from build123d import *

# Parameters (mm, degrees)
CROQUIS1_R              = 4
SALIENTE_EXTRUIR1_DEPTH = 12
CORTAR_EXTRUIR2_DEPTH   = 8
CORTAR_EXTRUIR3_START   = -2.5000001
CORTAR_EXTRUIR3_DEPTH   = 4.0000001


# Read off the part's stored shape, not the designer's step: Cortar-Extruir3
with BuildPart() as part:
    # Croquis1 → Saliente-Extruir1 (new body)
    with BuildSketch(Plane.XY):
        Circle(CROQUIS1_R)
    extrude(amount=SALIENTE_EXTRUIR1_DEPTH)

    # Croquis1<5> → Cortar-Extruir2 (cut)
    with BuildSketch(Plane.XY):
        with BuildLine():
            Line((-1.322875656, 1.5), (1.322875656, 1.5))
            ThreePointArc((1.322875656, 1.5), (0, -2), (-1.322875656, 1.5))
        make_face()
    extrude(amount=CORTAR_EXTRUIR2_DEPTH, mode=Mode.SUBTRACT)

    # Cortar-Extruir3 outline → Cortar-Extruir3 (cut)
    with BuildSketch(Plane.XZ.offset(-1.5).offset(CORTAR_EXTRUIR3_START)):
        with BuildLine():
            ThreePointArc((2, 5), (0, 7), (-2, 5))
            Line((-2, 5), (-2, 2.5))
            ThreePointArc((-2, 2.5), (0, 0.5), (2, 2.5))
            Line((2, 2.5), (2, 5))
        make_face()
    extrude(amount=CORTAR_EXTRUIR3_DEPTH, mode=Mode.SUBTRACT)


solid = part.part
Could you check a few things on this model? Use its own coordinates, in mm. A direction names the side the tool comes from. Coordinates: 2 decimals unless noted, no trailing zeros. Order: outer loops, then holes, each group sorted by start corner. A loop starts at its lowest first (then second) coordinate and runs counter-clockwise, first axis right, second up.
Q1. Suppose I cut it at A-A on x = 0. Please give me the cut outline in (y, z), and give its area (4 significant figures).
Q2. Suppose I cut it at B-B on y = 3. Please give me the cut outline in (x, z).
Q3. Thinking about a two-plate mould opening in X: for faces 4 (the flat face through (0, 0, 12)), 5 (the flat face through (0, 1.5, 0.3)), 6 (the cylindrical face through (-0.867, -3.905, 5.916)), which applies, released by +X, released by -X, zero draft, split by the parting line, or undercut?
Q4. Will these pins go through, and if not, where does the flat tip stop? pin 1 (1.2 mm diameter, centred on y = 1.5, z = 3, fed in from -X); pin 2 (1.2 mm diameter, centred on y = 1, z = 3.5, fed in from +X); pin 3 (1.5 mm diameter, centred on x = -2, z = 6, fed in from -Y).
Q5. Please list where these lines run through material, in increasing order: L1, parallel to Z at x = 0.75, y = 3.5; L2, parallel to Z at x = -0.75, y = 0; L3, parallel to X at y = -0.5, z = 5.25.
Q6. Suppose I cut it at C-C on z = 3.75. Please give me the cut outline in (x, y), and give its area (3 significant figures).
Q7. Which directions (+Z, -Z, +X, -X, +Y, -Y) give clear straight access to the entire face, cutting with the end or side of a thin tool? Please do faces 1 (the flat face through (0, 2, 0)), 2 (the flat face through (0, 0, 8)), 3 (the flat face through (-2, 2, 4)).
Q8. Suppose I cut it at D-D on y = 0.25. Please give me the cut outline in (x, z).
Answer:
1. outline: (-4, 0) - (-2, 0) - (-2, 8) - (1.5, 8) - (1.5, 7) - (4, 7) - (4, 12) - (-4, 12) - close; (1.5, 0) - (4, 0) - (4, 0.5) - (1.5, 0.5) - close
1. area: 51.75 mm2
2. outline: (-2.65, 0) - (2.65, 0) - (2.65, 12) - (-2.65, 12) - close; hole (-2, 2.5) arc R2 ccw to (2, 2.5) - (2, 5) arc R2 ccw to (-2, 5) - close
3. face 4: zero draft
3. face 5: undercut
3. face 6: split by the parting line
4. pin 1: stops at x = -3.9
4. pin 2: stops at x = 3.98
4. pin 3: stops at y = -3.8
5. L1: z = 0 to 0.65, 6.85 to 12
5. L2: z = 8 to 12
5. L3: x = -3.97 to -1.94, 1.94 to 3.97
6. outline: (-2, 0) - (-2, 3.46) arc R4 ccw (long way) to (2, 3.46) - (2, 0) arc R2 cw to start
6. area: 28.7 mm2
7. face 1: -Z, +X, -X, +Y, -Y
7. face 2: -Z
7. face 3: +Y
8. outline: (-3.99, 0) - (-1.98, 0) - (-1.98, 2.25) arc R2 cw to (-2, 2.5) - (-2, 5) arc R2 cw to (-1.98, 5.25) - (-1.98, 8) - (1.98, 8) - (1.98, 5.25) arc R2 cw to (2, 5) - (2, 2.5) arc R2 cw to (1.98, 2.25) - (1.98, 0) - (3.99, 0) - (3.99, 12) - (-3.99, 12) - close
